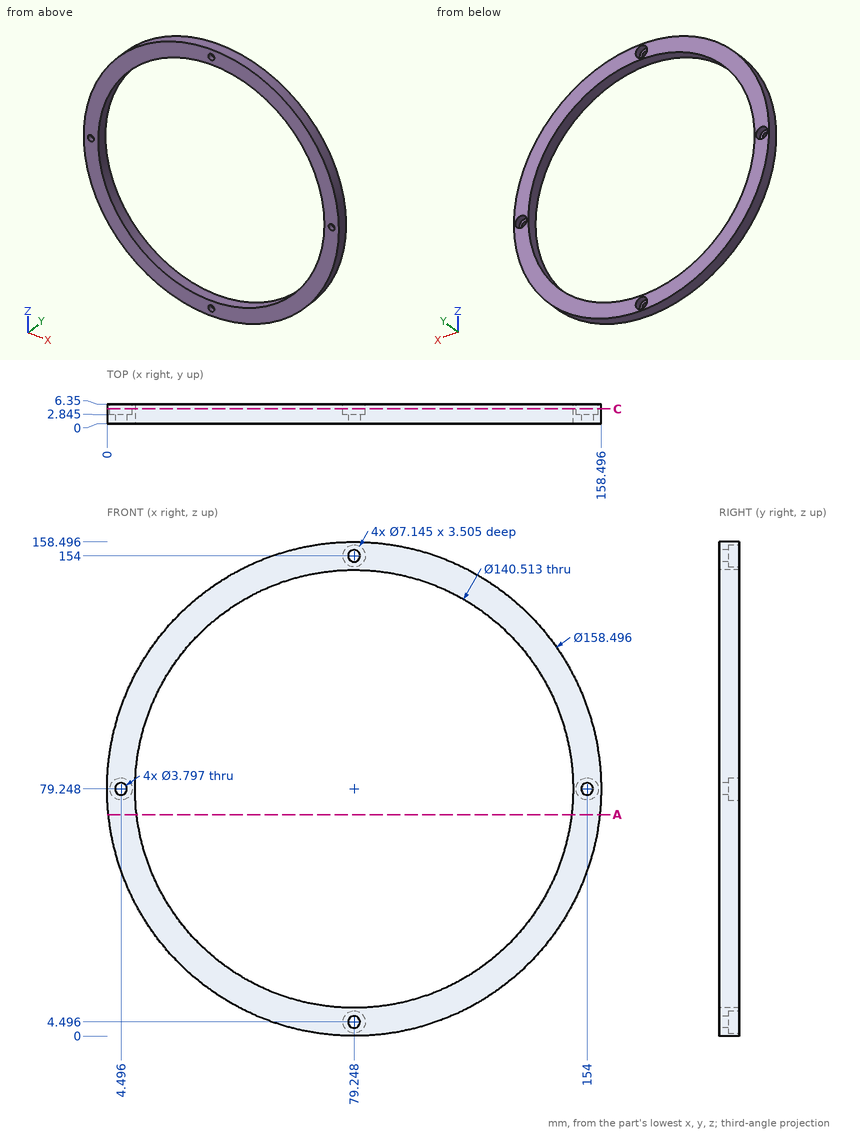
Source: three-view drawing plus pictorial views. Frame: mm from the lowest corner of the part. Give positions to 0.01 mm unless a question says otherwise; leave off trailing zeros. Write each loop counter-clockwise with the first axis right and the second up, starting at its lowest first coordinate (ties: lowest second). Pieces come first, ordered by that corner, then holes. Notation, with made-up numbers: (3, 38.25) -> (30, 38.25) arc R19 ccw to (30, 54.25) -> close; hole circle Ø6 at (4, -39.5). An arc over 180 degrees is marked (long way). Write item = value, one per line.
Q1. Cut plane C-C on y = 4.75. Return loops of the section in (x, z) (1 decimal), then the cut area to 3 significant figures.
Here are the results:
outline = circle Ø158.5 at (79.2, 79.2); hole circle Ø7.1 at (4.5, 79.2); hole circle Ø140.5 at (79.2, 79.2); hole circle Ø7.1 at (79.2, 4.5); hole circle Ø7.1 at (79.2, 154); hole circle Ø7.1 at (154, 79.2)
area = 4,060 mm²
Q2. First-contact query: pin 1 (2 mm diameter, centred on x = 3, z = 81, fed in from +Y) (1 decimal); pin 2 (3 mm diameter, centred on y = 4, z = 132.5, fed in from +X) (1 decimal); pin 3 (2 mm diameter, centred on x = 87, y = 2.5, fed in from +Z). Flat tips, straight axial feed; report the tip coordinate or a pass-through.
Here are the results:
pin_1 = 2.8
pin_2 = 139.3
pin_3 = 158.21
Q3. Line query: line 1 (X direction, y = 5.75, z = 78); line 2 (Z direction, x = 58, y = 4.5) (1 decimal); line 3 (Z direction, x = 39.5, y = 2.5). Output: solid intervals per line, ascending. Write a range as from..to.
Here are the results:
line_1 = 0.01..1.15, 7.84..9, 149.49..150.65, 157.35..158.49
line_2 = 2.9..12.3, 146.2..155.6
line_3 = 10.69..21.32, 137.18..147.81
Q4. Cut plane A-A on z = 71. Return loops of the section in (x, y), then the cut area to 3 significant figures.
Here are the results:
outline = (0.43, 0) -> (9.48, 0) -> (9.48, 6.35) -> (0.43, 6.35) -> close; (149.02, 0) -> (158.07, 0) -> (158.07, 6.35) -> (149.02, 6.35) -> close
area = 115 mm²
